```python
from build123d import *

# Parameters (mm, degrees)
F1_R     = 17
F1_R_2   = 15.5
F2_DEPTH = 115
F3_R     = 17
F4_DEPTH = 2
F5_R     = 15.25
F6_DEPTH = 10


with BuildPart() as f2:
    # F1 (on offset) → F2 (new body)
    with BuildSketch(Plane.XY.offset(222)):
        Circle(F1_R)
        Circle(F1_R_2, mode=Mode.SUBTRACT)
    extrude(amount=F2_DEPTH)

    # F3 (on offset) → F4 (join)
    with BuildSketch(Plane.XY.offset(222)):
        Circle(F3_R)
    extrude(amount=F4_DEPTH)

    # F5 (on face) → F6 (join)
    with BuildSketch(Plane(origin=(0, 0, 222), x_dir=(1, 0, 0), z_dir=(0, 0, -1))):
        Circle(F5_R)
    extrude(amount=F6_DEPTH)


solid = f2.part
```
Design review of the part built by this model. Coordinates are the model's own, in mm. A direction names the side the tool comes from. Give positions to 0.01 mm unless a question says otherwise; leave off trailing zeros. Write each loop counter-clockwise with the first axis right and the second up, starting at its lowest first coordinate (ties: lowest second). Pieces come first, ordered by that corner, then holes. Notation, with made-up numbers: (30.5, 2) - (44.5, 2) arc R15 cw to (44.5, 24) - close; hole circle Ø7 at (22.25, 71). An arc over 180 degrees is marked (long way). Return JSON: item names as keys, results as strings. Group by question number.
(1) To check wall thickness, follow probe 1 along Y at (x, z) = (0, 300); probe 2 along Z at (x, y) = (10, -7); probe 3 along X at (y, z) = (12, 303). State the ranges of each line that lie inside material, in increasing order.
(2) We need section A-A, the plane x = 0. Give the boundary of the cut face in (y, z).
(3) Machinability: for faces 4 (the flat face through (0, 0, 224)), 5 (the cylindrical face through (-12.1, 9.28, 217.07)), 6 (the flat face through (0, 0, 212)), which of the approach directions +Z, -Z, +X, -X, +Y, -Y give a long, thin tool a straight path to every point of the face, cutting with its end or side? Answer none if there is none.
(4) Mouldability with a two-part tool opening along X and no side actions: class faces 1 (the flat face through (-13, -9, 222)), 2 (the cylindrical face through (-2.018, 15.368, 279.709)), 3 (the cylindrical face through (9.139, 14.334, 278.695)) as +X half, -X half, draft (parallel to the pull), parting line (faces both ways), or undercut.
(5) We need section B-B, the plane z = 306.5. Give the boundary of the cut face in (x, y).
(6) Insertion check: pin 1 (6 mm diameter, centred on x = 5, z = 283.5, fed in from -Y); pin 2 (1 mm diameter, centred on y = 12, z = 276, fed in from +X); pin 3 (8 mm diameter, centred on y = -13, z = 302.5, fed in from -X). Each pin has a flat end and moves straight along its axis. Give the tip position at first contact, or say it passes through.
(7) We need section C-C, the plane y = 12. Give the boundary of the cut face in (x, z).
Reported:
{
 "1": {"probe 1": "y = -17 to -15.5, 15.5 to 17", "probe 2": "z = 212 to 224", "probe 3": "x = -12.04 to -9.81, 9.81 to 12.04"},
 "2": {"outline": "(-17, 222) - (-15.25, 222) - (-15.25, 212) - (15.25, 212) - (15.25, 222) - (17, 222) - (17, 337) - (15.5, 337) - (15.5, 224) - (-15.5, 224) - (-15.5, 337) - (-17, 337) - close"},
 "3": {"face 4": "+Z", "face 5": "-Z", "face 6": "-Z, +X, -X, +Y, -Y"},
 "4": {"face 1": "draft", "face 2": "undercut", "face 3": "parting line"},
 "5": {"outline": "circle Ø34 at (0, 0); hole circle Ø31 at (0, 0)"},
 "6": {"pin 1": "stops at y = -16.88", "pin 2": "stops at x = 12.52", "pin 3": "stops at x = -14.42"},
 "7": {"outline": "(-12.04, 222) - (-9.41, 222) - (-9.41, 212) - (9.41, 212) - (9.41, 222) - (12.04, 222) - (12.04, 337) - (9.81, 337) - (9.81, 224) - (-9.81, 224) - (-9.81, 337) - (-12.04, 337) - close"}
}
